Check sheet for the modelled part. Datum: model origin and axes. Units: mm. A direction names the side the tool comes from. Round coordinates to 2 decimals unless told otherwise and drop trailing zeros. Loops run counter-clockwise (first coordinate to the right, second up) from the corner with the lowest first, then second, coordinate; pieces in that order, holes last. Notation, with made-up numbers: (-15, -0.5) - (29, -0.5) arc R21 ccw to (29, 28.5) - close; hole circle Ø7 at (52, 42). An arc over 180 degrees is marked (long way). Put each result on its own line as item: value. Start each with the question number.
Item 1: Section check A-A, the plane z = -13.25. Record the cut outline in (x, y), and give its area (3 significant figures).
Item 2: Material ranges on line 1 along X through (y, z) = (-115.5, -14); line 2 along Y through (x, z) = (211, -8); line 3 along Y through (x, z) = (232.5, -15.75), recorded low to high.
Item 3: Section check C-C, the plane y = -62. Record the cut outline in (x, z), and give its area (3 significant figures).
Item 4: Section check B-B, the plane y = -312. Record the cut outline in (x, z).
Item 5: Tool access check on faces 5 (the flat face through (25.4, -206, -13)), 6 (the flat face through (165, -330.2, -13)). Record the directions out of +Z, -Z, +X, -X, +Y, -Y that give a thin tool (end or side, any length) a straight path to the whole face; none if there is none.
Item 6: Draft check along Y on faces 1 (the flat face through (203, -355.6, -13)), 2 (the flat face through (206, -25.4, -13)), 3 (the flat face through (280, -201, -25.4)), 4 (the flat face through (201, -381, -13)). Enter one of: pulls with the +Y half, pulls with the -Y half, needs draft (parallel to the pull), parting line crosses it, or undercut.
Autodesk Inventor part; units mm, degrees
ref_plane "YZ Plane" through (0, 0, 0) normal (1, 0, 0) x (0, 1, 0)
ref_plane "XZ Plane" through (0, 0, 0) normal (0, 1, 0) x (-1, 0, 0)
ref_plane "XY Plane" through (0, 0, 0) normal (0, 0, 1) x (1, 0, 0)
sketch "Sketch1" plane through (0, 0, 0) normal (0, 0, 1) x (1, 0, 0)
  line L0 (0, 0) -> (812.8, 0) construction
  line L1 (812.8, 0) -> (812.8, -406.4) construction
  line L2 (812.8, -406.4) -> (0, -406.4) construction
  line L3 (0, -406.4) -> (0, 0) construction
  line L4 (0, 0) -> (406.4, 0)
  line L5 (406.4, 0) -> (406.4, -25.4)
  line L6 (406.4, -25.4) -> (0, -25.4)
  line L7 (0, -25.4) -> (0, 0)
  line L8 (406.4, -25.4) -> (381, -25.4)
  line L9 (381, -25.4) -> (381, -406.4)
  line L10 (381, -406.4) -> (406.4, -406.4)
  line L11 (406.4, -406.4) -> (406.4, -25.4)
  line L12 (381, -406.4) -> (0, -406.4)
  line L13 (0, -406.4) -> (0, -381)
  line L14 (0, -381) -> (381, -381)
  line L15 (381, -381) -> (381, -406.4)
  line L16 (0, -381) -> (25.4, -381)
  line L17 (25.4, -381) -> (25.4, -25.4)
  line L18 (25.4, -25.4) -> (0, -25.4)
  line L19 (0, -25.4) -> (0, -381)
  dimension "d1" = 812.8
  dimension "d5" = 406.4
  dimension "d6" = 25.4
  dimension "d7" = 25.4
  dimension "d8" = 381
  dimension "d9" = 381
  dimension "d10" = 25.4
  dimension "d11" = 25.4
extrude "Extrusion1" add sketch "Sketch1" against normal blind 25.4 contours L6 L9 L14 L17
sketch "Sketch3" plane through (0, 0, 0) normal (0, 0, 1) x (1, 0, 0)
  line L0 (-406.4, 0) -> (406.4, 0) construction
  line L1 (406.4, 0) -> (406.4, -406.4) construction
  line L2 (406.4, -406.4) -> (-406.4, -406.4) construction
  line L3 (-406.4, -406.4) -> (-406.4, 0) construction
  line L4 (406.4, 0) -> (406.4, -406.4)
  line L5 (381, -381) -> (25.4, -381)
  line L6 (203.2, -381) -> (203.2, -355.6)
  line L7 (203.2, -355.6) -> (254, -355.6)
  line L8 (254, -355.6) -> (254, -50.8)
  line L9 (254, -50.8) -> (152.4, -50.8)
  line L10 (152.4, -50.8) -> (152.4, -355.6)
  line L11 (152.4, -355.6) -> (203.2, -355.6)
  point P0 (0, 0)
  dimension "d36" = 812.8
  dimension "d45" = 25.4
  dimension "d46" = 50.8
  dimension "d47" = 304.8
  dimension "d48" = 101.6
extrude "Extrusion3" cut sketch "Sketch3" against normal blind 25.4
sketch "Sketch4" plane through (0, 0, 0) normal (0, 0, 1) x (1, 0, 0)
  line L0 (254, -50.8) -> (152.4, -50.8)
  line L1 (152.4, -50.8) -> (177.8, -50.8)
  line L2 (177.8, -50.8) -> (177.8, -76.2)
  line L3 (177.8, -76.2) -> (152.4, -76.2)
  line L4 (152.4, -76.2) -> (152.4, -50.8)
  line L5 (254, -50.8) -> (228.6, -50.8)
  line L6 (228.6, -50.8) -> (228.6, -76.2)
  line L7 (228.6, -76.2) -> (254, -76.2)
  line L8 (254, -76.2) -> (254, -50.8)
  line L9 (152.4, -355.6) -> (254, -355.6)
  line L10 (152.4, -355.6) -> (177.8, -355.6)
  line L11 (177.8, -355.6) -> (177.8, -330.2)
  line L12 (177.8, -330.2) -> (152.4, -330.2)
  line L13 (152.4, -330.2) -> (152.4, -355.6)
  line L14 (254, -355.6) -> (228.6, -355.6)
  line L15 (228.6, -355.6) -> (228.6, -330.2)
  line L16 (228.6, -330.2) -> (254, -330.2)
  line L17 (254, -330.2) -> (254, -355.6)
  point P0 (0, 0)
  dimension "d51" = 25.4
  dimension "d52" = 25.4
  dimension "d53" = 25.4
  dimension "d54" = 25.4
  dimension "d55" = 25.4
  dimension "d56" = 25.4
  dimension "d57" = 25.4
  dimension "d58" = 25.4
extrude "Extrusion4" add sketch "Sketch4" against normal blind 25.4
properties part number "JukeBox Top Panel"
Check result:
1. outline: (25.4, -381) - (381, -381) - (381, -25.4) - (25.4, -25.4) - close; hole (152.4, -330.2) - (177.8, -330.2) - (177.8, -355.6) - (228.6, -355.6) - (228.6, -330.2) - (254, -330.2) - (254, -76.2) - (228.6, -76.2) - (228.6, -50.8) - (177.8, -50.8) - (177.8, -76.2) - (152.4, -76.2) - close
1. area: 98,100 mm²
2. line 1: 25.4 to 152.4, 254 to 381
2. line 2: -381 to -355.6, -50.8 to -25.4
2. line 3: -381 to -330.2, -76.2 to -25.4
3. outline: (25.4, -25.4) - (177.8, -25.4) - (177.8, 0) - (25.4, 0) - close; (228.6, -25.4) - (381, -25.4) - (381, 0) - (228.6, 0) - close
3. area: 7,740 mm²
4. outline: (25.4, -25.4) - (152.4, -25.4) - (152.4, 0) - (25.4, 0) - close; (254, -25.4) - (381, -25.4) - (381, 0) - (254, 0) - close
5. face 5: +Z, -Z, -X, +Y, -Y
5. face 6: +Z, -Z
6. face 1: undercut
6. face 2: pulls with the +Y half
6. face 3: needs draft
6. face 4: pulls with the -Y half
